Can you work these out from the model? Positions are in its coordinate system, mm. A direction names the side the tool comes from. Give positions to 0.01 mm unless a question says otherwise; leave off trailing zeros. Loops run counter-clockwise (first coordinate to the right, second up) from the corner with the lowest first, then second, coordinate; pieces in that order, holes last. Notation, with made-up numbers: (-12, -13) - (28, -13) arc R33 ccw to (28, 19) - close; hole circle Ø7 at (27.5, -4.75). An arc over 180 degrees is marked (long way). Write item = value, one per line.
from build123d import *

# Parameters (mm, degrees)
F1_DEPTH = 38.1
F2_W     = 88.9
F2_H     = 101.6
F3_DEPTH = 19.05
F4_W     = 88.9
F4_H     = 6.35
F5_DEPTH = 38.1
F8_R     = 5.08


with BuildPart() as f1:
    # F0 (on Top) → F1 (new body)
    with BuildSketch(Plane.XY):
        Polygon((-31.983944577, 23.2039450469), (-31.983944577, -40.2960549531), (56.916055423, -40.2960549531), (56.916055423, -2.1960549531), align=None)
    extrude(amount=F1_DEPTH)

    # F2 (on face) → F3 (join)
    with BuildSketch(Plane.XY.offset(38.1)):
        with Locations((12.466055423, 10.5039450469)):
            Rectangle(F2_W, F2_H)
    extrude(amount=F3_DEPTH)

    # F4 (on face) → F5 (join)
    with BuildSketch(Plane.XY.offset(57.15)):
        with Locations((12.466055423, 58.1289450469)):
            Rectangle(F4_W, F4_H)
    extrude(amount=F5_DEPTH)


with BuildPart() as f6_1:
    # F6: instance of F1
    add(f1.part.mirror(Plane.XY))

    # F8
    f8_edges = [f6_1.edges().sort_by_distance(p)[0] for p in [
        (56.916055, 7.328945, -57.15),
        (-31.983945, 7.328945, -57.15),
        (56.916055, 58.128945, -95.25),
        (-31.983945, 58.128945, -95.25),
    ]]
    fillet(f8_edges, radius=F8_R)


solid = f6_1.part
Q1. I need wall thicknesses on L1, parallel to Z at x = -9, y = 23.5; L2, parallel to Z at x = 16.5, y = -3.5; L3, parallel to Y at x = 31.5, z = -74.5. Which ranges of each line are inside material? Lowest first, please.
Output:
L1 = -57.15 to -38.1
L2 = -57.15 to 0
L3 = 54.95 to 61.3
Q2. For pin 1 (19 mm diameter, centred on x = 16, y = 36.5, fed in from +Z); pin 2 (6 mm diameter, centred on x = -21.5, y = 39, fed in from -Z); pin 3 (8 mm diameter, centred on x = -8.5, z = -28.5, fed in from +Y), each with a flat end and sliding along its axis, tell me the tip position at first contact or that it passes through.
Output:
pin_1 = -38.1
pin_2 = -57.15
pin_3 = 17.64
Q3. Imagine slicing it at D-D, the plane y = -26.5. Write out the boundary of the cut face in (x, z).
Output:
outline = (-31.98, -52.07) arc R5.08 ccw to (-26.9, -57.15) - (51.84, -57.15) arc R5.08 ccw to (56.92, -52.07) - (56.92, 0) - (-31.98, 0) - close
Q4. Which directions (+Z, -Z, +X, -X, +Y, -Y) give clear straight access to the entire face, cutting with the end or side of a thin tool? Please do faces 1 (the cylindrical face through (-30.54, 8, -55.62)), 2 (the flat face through (13.088, 10.326, -18.783)), 3 (the cylindrical face through (55.39, 8, -55.7)), 4 (the flat face through (12, 8, -57.15)).
Output:
face_1 = -Z, -X, -Y
face_2 = +Z, +X, +Y
face_3 = -Z, +X, -Y
face_4 = -Z, +X, -X, -Y
Q5. Imagine slicing it at C-C, the plane z = -6.5. Write out the boundary of the cut face in (x, y), then the cut area to 3 significant figures.
Output:
outline = (-31.98, -40.3) - (56.92, -40.3) - (56.92, -2.2) - (-31.98, 23.2) - close
area = 4,520 mm2
Q6. Imagine slicing it at A-A, the plane y = 25. Write out the boundary of the cut face in (x, z).
Output:
outline = (-31.98, -52.07) arc R5.08 ccw to (-26.9, -57.15) - (51.84, -57.15) arc R5.08 ccw to (56.92, -52.07) - (56.92, -38.1) - (-31.98, -38.1) - close
Q7. Imagine slicing it at B-B, the plane x = -1. Write out the boundary of the cut face in (y, z), then the cut area to 3 significant figures.
Output:
outline = (-40.3, -57.15) - (54.95, -57.15) - (54.95, -95.25) - (61.3, -95.25) - (61.3, -38.1) - (14.35, -38.1) - (14.35, 0) - (-40.3, 0) - close
area = 4,260 mm2
